Geometry: final body of the model. Coordinates: model frame, mm. A direction names the side the tool comes from. Coordinates: 2 decimals unless noted, no trailing zeros. Order: outer loops, then holes, each group sorted by start corner. A loop starts at its lowest first (then second) coordinate and runs counter-clockwise, first axis right, second up. Notation, with made-up numbers: M 14.25,-8.5 L 50.25,-8.5 A20 cw 50.25,23.5 Z; hole C 18.25,-6.75 d7. An arc over 180 degrees is marked long. Write item = value, one per line. Start each with the question number.
Autodesk Inventor part; units mm, degrees
ref_plane "YZ Plane" through (0, 0, 0) normal (1, 0, 0) x (0, 1, 0)
ref_plane "XZ Plane" through (0, 0, 0) normal (0, 1, 0) x (-1, 0, 0)
ref_plane "XY Plane" through (0, 0, 0) normal (0, 0, 1) x (1, 0, 0)
sketch "Sketch1" plane through (0, 0, 0) normal (0, 0, 1) x (1, 0, 0)
  point P0 (0, 0)
sketch "Sketch2" plane through (0, 0, 0) normal (0, 0, 1) x (1, 0, 0)
  line L0 (-22.3056, -24.3056) -> (22.3056, -24.3056)
  line L1 (24.3056, -22.3056) -> (24.3056, 22.3056)
  line L2 (22.3056, 24.3056) -> (-22.3056, 24.3056)
  line L3 (-24.3056, 22.3056) -> (-24.3056, -22.3056)
  line L4 (-24.3056, -24.3056) -> (24.3056, 24.3056) construction
  line L5 (24.3056, -24.3056) -> (-24.3056, 24.3056) construction
  line L6 (-36.8889, -38.8889) -> (36.8889, -38.8889)
  line L7 (38.8889, -36.8889) -> (38.8889, 36.8889)
  line L8 (36.8889, 38.8889) -> (-36.8889, 38.8889)
  line L9 (-38.8889, 36.8889) -> (-38.8889, -36.8889)
  line L10 (-38.8889, -38.8889) -> (38.8889, 38.8889) construction
  line L11 (38.8889, -38.8889) -> (-38.8889, 38.8889) construction
  arc A0 (-36.8889, 38.8889) -> (-38.8889, 36.8889) centre (-36.8889, 36.8889) ccw
  arc A1 (38.8889, 36.8889) -> (36.8889, 38.8889) centre (36.8889, 36.8889) ccw
  arc A2 (36.8889, -38.8889) -> (38.8889, -36.8889) centre (36.8889, -36.8889) ccw
  arc A3 (-38.8889, -36.8889) -> (-36.8889, -38.8889) centre (-36.8889, -36.8889) ccw
  arc A4 (-24.3056, -22.3056) -> (-22.3056, -24.3056) centre (-22.3056, -22.3056) ccw
  arc A5 (22.3056, -24.3056) -> (24.3056, -22.3056) centre (22.3056, -22.3056) ccw
  arc A6 (24.3056, 22.3056) -> (22.3056, 24.3056) centre (22.3056, 22.3056) ccw
  arc A7 (-22.3056, 24.3056) -> (-24.3056, 22.3056) centre (-22.3056, 22.3056) ccw
  point P0 (0, 0)
  dimension "HL" = 48.6111
  dimension "d1" = 24.3056
  dimension "d2" = 77.7778
  dimension "d3" = 38.8889
  dimension "d4" = 2
extrude "Extrusion1" add sketch "Sketch2" along normal blind 15.5556
equation "\"d2\" = 1.6 * HL"
equation "\"d5\" = 0.32 * HL"
properties part number "Ram(Nästankvadratisk"
Item 1: Reachability of faces 4 (the cylindrical face through (38.287, 38.319, 7.669)), 5 (the flat face through (0, 24.306, 8)) from +Z, -Z, +X, -X, +Y, -Y: full face, straight path, thin tool, end or side. Return the list, or none.
Item 2: Material intervals for probe 1 along X at (y, z) = (-10.5, 14.25); probe 2 along Y at (x, z) = (24, 3), sorted ascending. Write a range as [from, to].
Item 3: Section query A-A on y = 7.5. Output: boundary loops of the cut face in (x, z), and give its area (3 significant figures).
Item 4: Section query C-C on z = 12. Output: boundary loops of the cut face in (x, y), and give its area (3 significant figures).
Item 5: Draft query along Y for faces 1 (the flat face through (-38.889, 1, 8)), 2 (the cylindrical face through (-23.74, 23.7, 7.67)), 3 (the cylindrical face through (-38.319, 38.287, 7.669)). Return one class per face: pulls with the +Y half, pulls with the -Y half, needs draft (parallel to the pull), parting line crosses it, or undercut.
Ans:
q1.face_4 = +Z, -Z, +X, +Y
q1.face_5 = +Z, -Z
q2.probe_1 = [-38.89, -24.31], [24.31, 38.89]
q2.probe_2 = [-38.89, -23.37], [23.37, 38.89]
q3.outline = M -38.89,0 L -24.31,0 L -24.31,15.56 L -38.89,15.56 Z; M 24.31,0 L 38.89,0 L 38.89,15.56 L 24.31,15.56 Z
q3.area = 454 mm^2
q4.outline = M -38.89,-36.89 A2 ccw -36.89,-38.89 L 36.89,-38.89 A2 ccw 38.89,-36.89 L 38.89,36.89 A2 ccw 36.89,38.89 L -36.89,38.89 A2 ccw -38.89,36.89 Z; hole M -24.31,-22.31 A2 ccw -22.31,-24.31 L 22.31,-24.31 A2 ccw 24.31,-22.31 L 24.31,22.31 A2 ccw 22.31,24.31 L -22.31,24.31 A2 ccw -24.31,22.31 Z
q4.area = 3,690 mm^2
q5.face_1 = needs draft
q5.face_2 = undercut
q5.face_3 = pulls with the +Y half
